```python
from build123d import *

# Parameters (mm, degrees)
SKETCH1_R           = 3.17
SKETCH1_R_2         = 11.1
SKETCH1_R_3         = 2
BOSS_EXTRUDE2_DEPTH = 2


with BuildPart() as part:
    # Sketch1 → Boss-Extrude2 (new body)
    with BuildSketch(Plane(origin=(0, 0, 0), x_dir=(0, 0, -1), z_dir=(1, 0, 0))):
        with BuildLine():
            Line((47.801233781, -63.131130768), (47.801233781, -21.131130768))
            Line((47.801233781, -21.131130768), (37.801233781, -21.131130768))
            Line((37.801233781, -21.131130768), (37.801233781, -20.131130768))
            ThreePointArc((37.801233781, -20.131130768), (37.508340562, -19.424023986), (36.801233781, -19.131130768))
            Line((36.801233781, -19.131130768), (23.801233781, -19.131130768))
            ThreePointArc((23.801233781, -19.131130768), (23.094127, -19.424023986), (22.801233781, -20.131130768))
            Line((22.801233781, -20.131130768), (22.801233781, -21.131130768))
            Line((22.801233781, -21.131130768), (17.801233781, -21.131130768))
            Line((17.801233781, -21.131130768), (17.801233781, 23.868869232))
            Line((17.801233781, 23.868869232), (9.55072491, 23.868869232))
            Line((9.55072491, 23.868869232), (9.55072491, 24.868869232))
            ThreePointArc((9.55072491, 24.868869232), (9.257831691, 25.575976014), (8.55072491, 25.868869232))
            Line((8.55072491, 25.868869232), (-29.948257347, 25.868869232))
            ThreePointArc((-29.948257347, 25.868869232), (-30.655364129, 25.575976014), (-30.948257347, 24.868869232))
            Line((-30.948257347, 24.868869232), (-30.948257347, 23.868869232))
            Line((-30.948257347, 23.868869232), (-34.398766219, 23.868869232))
            Line((-34.398766219, 23.868869232), (-34.398766219, 15.868869232))
            Line((-34.398766219, 15.868869232), (-36.398766219, 15.868869232))
            Line((-36.398766219, 15.868869232), (-36.398766219, 23.868869232))
            Line((-36.398766219, 23.868869232), (-42.198766219, 23.868869232))
            Line((-42.198766219, 23.868869232), (-42.198766219, -63.131130768))
            Line((-42.198766219, -63.131130768), (-30.948257347, -63.131130768))
            Line((-30.948257347, -63.131130768), (-30.948257347, -64.131130768))
            ThreePointArc((-30.948257347, -64.131130768), (-30.655364129, -64.838237549), (-29.948257347, -65.131130768))
            Line((-29.948257347, -65.131130768), (27.55072491, -65.131130768))
            ThreePointArc((27.55072491, -65.131130768), (28.257831691, -64.838237549), (28.55072491, -64.131130768))
            Line((28.55072491, -64.131130768), (28.55072491, -63.131130768))
            Line((28.55072491, -63.131130768), (47.801233781, -63.131130768))
        make_face()
        with Locations((-26.398766219, -19.631130768)):
            Circle(SKETCH1_R, mode=Mode.SUBTRACT)
        with Locations((29.515713155, -45.631130768)):
            Circle(SKETCH1_R_2, mode=Mode.SUBTRACT)
        with Locations((16.515713155, -32.631130768)):
            Circle(SKETCH1_R_3, mode=Mode.SUBTRACT)
        with Locations((42.515713155, -32.631130768)):
            Circle(SKETCH1_R_3, mode=Mode.SUBTRACT)
        with Locations((42.515713155, -58.631130768)):
            Circle(SKETCH1_R_3, mode=Mode.SUBTRACT)
        with Locations((16.515713155, -58.631130768)):
            Circle(SKETCH1_R_3, mode=Mode.SUBTRACT)
        with Locations((1.558473468, -32.631130768)):
            Circle(SKETCH1_R, mode=Mode.SUBTRACT)
    extrude(amount=BOSS_EXTRUDE2_DEPTH)


solid = part.part
```
Input: part model. Units: mm. Frame: model coordinates. A direction names the side the tool comes from. Give positions to 0.01 mm unless a question says otherwise; leave off trailing zeros. Order: outer loops, then holes, each group sorted by start corner. A loop starts at its lowest first (then second) coordinate and runs counter-clockwise, first axis right, second up. Notation, with made-up numbers: M 88.25,-14 L 138.25,-14 A16 ccw 138.25,10 Z; hole C 85.25,30.5 d3. An arc over 180 degrees is marked long. One line per question, with ' | ' between items.
1) Section B-B on y = -18. Output: boundary loops of the cut face in (x, z).
Filled in:
outline: M 0,-17.8 L 2,-17.8 L 2,23.68 L 0,23.68 Z; M 0,29.12 L 2,29.12 L 2,42.2 L 0,42.2 Z
2) Section D-D on x = 0.65. State how many separate pieces and enclosed holes the cut face has, and give its area (3 significant figures).
Filled in:
separate pieces: 1 | enclosed holes: 7 | area: 6,190 mm2
3) Ray query, L1, parallel to Z at x = 0.65, y = -59.5; L2, parallel to Z at x = 1.55, y = 18.5; L3, parallel to Z at x = 0.4, y = -33. Return the intervals inside material, ascending.
Filled in:
L1: z = -47.8 to -44.32, -40.71 to -18.32, -14.71 to 42.2 | L2: z = -17.8 to 34.4, 36.4 to 42.2 | L3: z = -47.8 to -44.48, -40.55 to -18.48, -14.55 to -4.71, 1.59 to 42.2
4) Section C-C on y = -6. Output: boundary loops of the cut face in (x, z).
Filled in:
outline: M 0,-17.8 L 2,-17.8 L 2,42.2 L 0,42.2 Z
5) Contact query for flat-ended pins moving along their axis: P1, Ø1, axis at x = 1.5, z = -36, coming from the -Y side; P2, Ø1.1, axis at x = 1.5, y = -20.5, coming from the -Z side. Output: stop coordinate, or through.
Filled in:
P1: stops at y = -63.13 | P2: stops at z = -37.8
6) Section A-A on z = -33.5. Output: boundary loops of the cut face in (x, y), and give its area (3 significant figures).
Filled in:
outline: M 0,-63.13 L 2,-63.13 L 2,-55.99 L 0,-55.99 Z; M 0,-35.27 L 2,-35.27 L 2,-19.13 L 0,-19.13 Z | area: 46.6 mm2
7) Draft query along Y for faces 1 (the face through (0.99, -31.28, -15.04)), 2 (the face through (1, 23.869, 39)), 3 (the face through (1, 20, 34.399)), 4 (the face through (1, -63.131, -38)). Return one class per face: pulls with the +Y half, pulls with the -Y half, needs draft (parallel to the pull), parting line crosses it, or undercut.
Filled in:
face 1: undercut | face 2: pulls with the +Y half | face 3: needs draft | face 4: pulls with the -Y half
8) Access query for faces 5 (the face through (1, 23.869, 33)), 6 (the face through (1, -19.131, -30)), 7 (the face through (1, 20, 36.399)). Directions: +Z, -Z, +X, -X, +Y, -Y. A direction counts if a zero-diameter tool reaches every point of the face in a straight line with its end or side. Return the directions, or none.
Filled in:
face 5: +Z, +X, -X, +Y | face 6: -Z, +X, -X, +Y | face 7: +X, -X, +Y
